Part model, mm, in its own coordinate system. Face numbers are marked on the shaded views. Give positions to 0.01 mm unless a question says otherwise; leave off trailing zeros. Write each loop counter-clockwise with the first axis right and the second up, starting at its lowest first coordinate (ties: lowest second). Pieces come first, ordered by that corner, then holes. Notation, with made-up numbers: (38, 41.5) - (73, 41.5) arc R8 ccw to (73, 51.5) - close; hole circle Ø4 at (43, 35). An arc over 180 degrees is marked (long way). Answer in a Markdown table with one row per item. Add a question column.
1. Band-saw the part on C-C on y = 1.5. Write the cut outline in (x, z).
2. Drop flat-ended pins along their axis: pin 1 Ø1.5 at (y, z) = (1, 2.5) entering from -X; pin 2 Ø3 at (x, z) = (-0.5, -1) entering from +Y. Give the stop position or say it passes through.
3. Band-saw the part on A-A on y = -0.1. Write the cut outline in (x, z), plus the area to 3 significant figures.
4. Probe line 1 along Z through (x, y) = (0, -0.45); line 2 along Z through (x, y) = (-1.25, 1.1); line 3 along X through (y, z) = (1.25, -0.25). List the from-to ranges inside material, lowest first.
5. Pull direction X, two halves, no side cores. Call the marked faces 1, 2 and 3: released by +X, released by -X, zero draft, split by the parting line, or undercut.
6. Band-saw the part on B-B on x = 0. Write the cut outline in (y, z), plus the area to 3 significant figures.
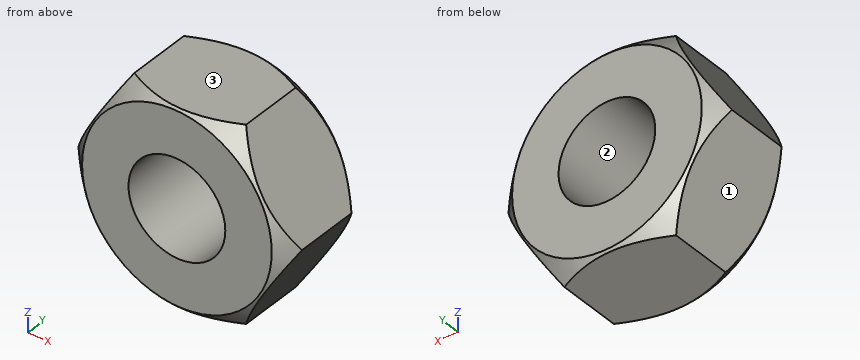
```python
from build123d import *

# Parameters (mm, degrees)
SKETCH1_R           = 2
BOSS_EXTRUDE1_DEPTH = 2


with BuildPart() as part:
    # Sketch1 → Boss-Extrude1 (new body, symmetric)
    with BuildSketch(Plane(origin=(0, 0, 0), x_dir=(1, 0, 0), z_dir=(0, 1, 0))):
        Polygon((2.309401077, 4), (-2.309401077, 4), (-4.618802154, 0), (-2.309401077, -4), (2.309401077, -4), (4.618802154, 0), align=None)
        Circle(SKETCH1_R, mode=Mode.SUBTRACT)
    extrude(amount=BOSS_EXTRUDE1_DEPTH, both=True)

    # Sketch2 → Cut-Revolve1 (revolve, cut)
    with BuildSketch(Plane.XY):
        Polygon((-4.618802154, 1.3), (-3.918802154, 2), (-4.618802154, 2), align=None)
    cut_revolve1 = revolve(axis=Axis((0, 0, 0), (0, 1, 0)), mode=Mode.SUBTRACT)

    # Mirror1: Cut-Revolve1 across plane
    add(cut_revolve1.mirror(Plane.ZX), mode=Mode.SUBTRACT)


solid = part.part
```
Values:
| question | item | result |
|---|---|---|
| 1 | outline | (-4.4, -0.37) - (-2.53, -3.63) arc R4.42 ccw to (-1.88, -4) - (1.88, -4) arc R4.42 ccw to (2.53, -3.63) - (4.4, -0.37) arc R4.42 ccw to (4.4, 0.37) - (2.53, 3.63) arc R4.42 ccw to (1.88, 4) - (-1.88, 4) arc R4.42 ccw to (-2.53, 3.63) - (-4.4, 0.37) arc R4.42 ccw to start; hole circle Ø4 at (0, 0) |
| 2 | pin 1 | stops at x = -3.61 |
| 2 | pin 2 | stops at y = 2 |
| 3 | outline | (-4.62, 0) - (-2.31, -4) - (2.31, -4) - (4.62, 0) - (2.31, 4) - (-2.31, 4) - close; hole circle Ø4 at (0, 0) |
| 3 | area | 42.9 mm² |
| 4 | line 1 | z = -4 to -2, 2 to 4 |
| 4 | line 2 | z = -4 to -1.56, 1.56 to 4 |
| 4 | line 3 | x = -4.47 to -1.98, 1.98 to 4.47 |
| 5 | face 1 | released by -X |
| 5 | face 2 | undercut |
| 5 | face 3 | zero draft |
| 6 | outline | (-2, -3.92) - (-1.92, -4) - (1.92, -4) - (2, -3.92) - (2, -2) - (-2, -2) - close; (-2, 2) - (2, 2) - (2, 3.92) - (1.92, 4) - (-1.92, 4) - (-2, 3.92) - close |
| 6 | area | 16.0 mm² |
